from build123d import *

# Parameters (mm, degrees)
SKETCH_1_R      = 85.5
SKETCH_1_R_2    = 50.5
EXTRUDE_1_DEPTH = 22
CHAMFER_1_SIZE  = 1
HOLE_WIZARD_1_D = 16


with BuildPart() as part:
    # 草图1 → 凸台-拉伸1 (new body)
    with BuildSketch(Plane(origin=(0, 0, 0), x_dir=(1, 0, 0), z_dir=(0, 1, 0))):
        with Locations(Location((0, 0, 0), (0, 0, 270))):
            Circle(SKETCH_1_R)
        with Locations(Location((0, 0, 0), (0, 0, 270))):
            Circle(SKETCH_1_R_2, mode=Mode.SUBTRACT)
    extrude(amount=EXTRUDE_1_DEPTH)

    # 倒角1
    chamfer_1_edges = [part.edges().sort_by_distance(p)[0] for p in [
        (0, 0, -85.5),
        (0, 22, -85.5),
        (0, 0, -50.5),
        (0, 22, -50.5),
    ]]
    chamfer(chamfer_1_edges, length=CHAMFER_1_SIZE)

    # 孔1 (through all)
    with Locations(Plane(origin=(0, 22, 0), x_dir=(1, 0, 0), z_dir=(0, 1, 0))):
        with Locations((46.315494168, 46.315494168), (65.5, 0), (46.315494168, -46.315494168), (0, -65.5), (-46.315494168, -46.315494168), (-65.5, 0), (-46.315494168, 46.315494168), (0, 65.5)):
            Hole(HOLE_WIZARD_1_D / 2)


solid = part.part
Build history of the part. All positions in model axes, mm. Round coordinates to 2 decimals unless told otherwise and drop trailing zeros. Write each loop counter-clockwise with the first axis right and the second up, starting at its lowest first coordinate (ties: lowest second). Pieces come first, ordered by that corner, then holes. Notation, with made-up numbers: M 9.25,70.25 L 22.25,70.25 A31 ccw 22.25,103.25 Z; hole C -5,70 d9. An arc over 180 degrees is marked long. Answer as a JSON object with one key per item and string values. Group by question number.
(1) Mould opens along X. For faces 1 (the cylindrical face through (84.772, 10.86, -11.13)), 2 (the cylindrical face through (1.041, 10.846, -73.432)), 3 (the flat face through (39, 22, 36)) say: pulls with the +X half, pulls with the -X half, needs draft (parallel to the pull), parting line crosses it, or undercut.
(2) Cut at C-C (y = 16). Give the number of separate pieces and of enclosed holes in the cut face, and give its area (3 significant figures).
(3) Cut at B-B (z = 0). Give the cut face in (x, y).
(4) Drill centre lines: L1, parallel to Z at x = 4.5, y = 9.75; L2, parallel to X at y = 18.25, z = -53; L3, parallel to Z at x = -41, y = 9.25. Where is each one in solid material? Low to high.
(5) Flat gauge pins, fed straight in: pin 1 (6 mm diameter, centred on x = -54, y = 13.5, fed in from +Z); pin 2 (14.5 mm diameter, centred on x = 46.32, z = -46.32, fed in from -Y) (3 decimals); pin 3 (12 mm diameter, centred on y = 14, z = 41.5, fed in from +X); pin 4 (12 mm diameter, centred on y = 12.5, z = -13.5, fed in from +X). Where does each tip first touch, or does it go through?
(6) Cut at A-A (x = 0). Give the cut face in (y, z), and give its area (3 significant figures).
Responses:
{
 "1": {"face 1": "parting line crosses it", "face 2": "undercut", "face 3": "needs draft"},
 "2": {"separate pieces": "1", "enclosed holes": "9", "area": "13,300 mm2"},
 "3": {"outline": "M -85.5,1 L -84.5,0 L -73.5,0 L -73.5,22 L -84.5,22 L -85.5,21 Z; M -57.5,0 L -51.5,0 L -50.5,1 L -50.5,21 L -51.5,22 L -57.5,22 Z; M 50.5,1 L 51.5,0 L 57.5,0 L 57.5,22 L 51.5,22 L 50.5,21 Z; M 73.5,0 L 84.5,0 L 85.5,1 L 85.5,21 L 84.5,22 L 73.5,22 Z"},
 "4": {"L1": "z = -85.38 to -72.11, -58.89 to -50.3, 50.3 to 58.89, 72.11 to 85.38", "L2": "x = -67.09 to -50.71, -41.92 to 41.92, 50.71 to 67.09", "L3": "z = -75.03 to -52.29, -40.34 to -29.48, 29.48 to 40.34, 52.29 to 75.03"},
 "5": {"pin 1": "stops at z = 68.62", "pin 2": "passes through", "pin 3": "stops at x = 77.78", "pin 4": "stops at x = 85.17"},
 "6": {"outline": "M 0,-84.5 L 1,-85.5 L 21,-85.5 L 22,-84.5 L 22,-73.5 L 0,-73.5 Z; M 0,-57.5 L 22,-57.5 L 22,-51.5 L 21,-50.5 L 1,-50.5 L 0,-51.5 Z; M 0,51.5 L 1,50.5 L 21,50.5 L 22,51.5 L 22,57.5 L 0,57.5 Z; M 0,73.5 L 22,73.5 L 22,84.5 L 21,85.5 L 1,85.5 L 0,84.5 Z", "area": "832 mm2"}
}
